Model file for the job. Use its own axes, mm. A direction names the side the tool comes from. Round coordinates to 2 decimals unless told otherwise and drop trailing zeros. Order: outer loops, then holes, each group sorted by start corner. A loop starts at its lowest first (then second) coordinate and runs counter-clockwise, first axis right, second up. Notation, with made-up numbers: (76, 88) - (110, 88) arc R20 cw to (110, 112) - close; hole circle Ø11 at (56.5, 32.25). An arc over 180 degrees is marked (long way). Answer as CSV lines item,"result". Start each with the question number.
1. Band-saw the part on A-A on z = 1.25. State how many separate pieces and enclosed holes the cut face has, then the cut area to 3 significant figures.
2. Pull direction X, two halves, no side cores. Call faces 3 (the face through (140.286, -328.814, 1.521)), 4 (the face through (108.17, -430.81, 1.52)), 5 (the face through (192.21, -358.5, 1.52)), 6 (the face through (154.939, -398.235, 1.479)): released by +X, released by -X, zero draft, split by the parting line, or undercut.
3. 3-axis set-ups, long thin cutter, end or side, ignore diameter. For faces 1 (the face through (120.483, -360.632, 1.521)), 2 (the face through (83.252, -416.399, 1.479)): which of +Z, -Z, +X, -X, +Y, -Y reach the whole face in a straight line?
4. Band-saw the part on C-C on y = -402. List the corners of the cut face in (x, z), then the cut area to 3 significant figures.
5. Wall check: line 1 along Y through (x, z) = (119, 0.8); line 2 along X through (y, z) = (-383.5, 0.8); line 3 along X through (y, z) = (-397, 0.65). Give the ranges that are in metal, low to high. Write a range as [from, to].
6. Band-saw the part on B-B on x = 168.5. List the corners of the cut face in (y, z).
7. Pin check, flat tips, straight feed: pin 1 Ø4 at (x, y) = (159.93, -323.72) entering from -Z; pin 2 Ø1 at (x, z) = (173.5, 1) entering from +Y. Stop position of each tip, or through.
```python
from build123d import *

# Parameters (mm, degrees)
EXTRUDE1_DEPTH     = 3
SKETCH2_R          = 2.65
CUT_EXTRUDE1_DEPTH = 5
SKETCH4_R          = 1.6
CUT_EXTRUDE3_DEPTH = 3


with BuildPart() as part:
    # Sketch1 → Extrude1 (new body)
    with BuildSketch(Plane.XY):
        Polygon((155.305831868, -303.657635717), (202.177156078, -355.648778874), (106.360004666, -442.030352657), (59.488680456, -390.0392095), align=None)
    extrude(amount=EXTRUDE1_DEPTH)

    # Sketch2 → Cut-Extrude1 (cut)
    with BuildSketch(Plane.XY.offset(3)):
        with Locations((135.499717478, -368.636757231)):
            Circle(SKETCH2_R)
    extrude(amount=-CUT_EXTRUDE1_DEPTH, mode=Mode.SUBTRACT)

    # Sketch4 → Cut-Extrude3 (cut)
    with BuildSketch(Plane.XY.offset(3)):
        with Locations((151.896067778, -314.809922875)):
            Circle(SKETCH4_R)
        with Locations((159.931151928, -323.722690273)):
            Circle(SKETCH4_R)
        with Locations((182.697223687, -348.975531235)):
            Circle(SKETCH4_R)
        with Locations((190.732307837, -357.888298634)):
            Circle(SKETCH4_R)
        with Locations((70.933528696, -387.79968974)):
            Circle(SKETCH4_R)
        with Locations((78.968612847, -396.712457139)):
            Circle(SKETCH4_R)
        with Locations((120.302950019, -405.225539455)):
            Circle(SKETCH4_R)
        with Locations((128.338034169, -414.138306853)):
            Circle(SKETCH4_R)
        with Locations((101.734684606, -421.965298101)):
            Circle(SKETCH4_R)
        with Locations((109.769768756, -430.878065499)):
            Circle(SKETCH4_R)
        with BuildLine():
            Line((80.285137719, -371.290679816), (134.509374605, -322.406165401))
            Line((134.509374605, -322.406165401), (146.227205658, -335.40395119))
            ThreePointArc((146.227205658, -335.40395119), (146.611102327, -336.485913681), (146.117495252, -337.522432634))
            Line((146.117495252, -337.522432634), (94.121450215, -384.398176011))
            ThreePointArc((94.121450215, -384.398176011), (93.039487724, -384.782072681), (92.002968771, -384.288465605))
            Line((92.002968771, -384.288465605), (80.285137719, -371.290679816))
        make_face()
        with BuildLine():
            ThreePointArc((154.253665546, -351.729600998), (150.369782899, -351.528465254), (150.168647155, -355.412347901))
            ThreePointArc((150.168647155, -355.412347901), (154.052529802, -355.613483645), (154.253665546, -351.729600998))
        make_face()
        with BuildLine():
            ThreePointArc((120.830787802, -381.861166562), (116.946905155, -381.660030818), (116.745769411, -385.543913464))
            ThreePointArc((116.745769411, -385.543913464), (120.629652058, -385.745049208), (120.830787802, -381.861166562))
        make_face()
    extrude(amount=-CUT_EXTRUDE3_DEPTH, mode=Mode.SUBTRACT)


solid = part.part
```
Reply:
1,separate pieces,"1"
1,enclosed holes,"13"
1,area,"7,490 mm2"
2,face 3,"released by -X"
2,face 4,"undercut"
2,face 5,"undercut"
2,face 6,"released by +X"
3,face 1,"+Z, -Z"
3,face 2,"+Z, -Z, -X, -Y"
4,outline,"(70.27, 0) - (150.76, 0) - (150.76, 3) - (70.27, 3) - close"
4,area,"241 mm2"
5,line 1,"y = [-430.64, -406.15], [-404.3, -386.44], [-380.96, -361.97]"
5,line 2,"x = [66.74, 91.29], [95.12, 116.05], [121.53, 171.28]"
5,line 3,"x = [65.76, 77.39], [80.54, 156.31]"
6,outline,"(-386.01, 0) - (-318.29, 0) - (-318.29, 3) - (-386.01, 3) - close"
7,pin 1,"stops at z = 0"
7,pin 2,"stops at y = -323.28"
